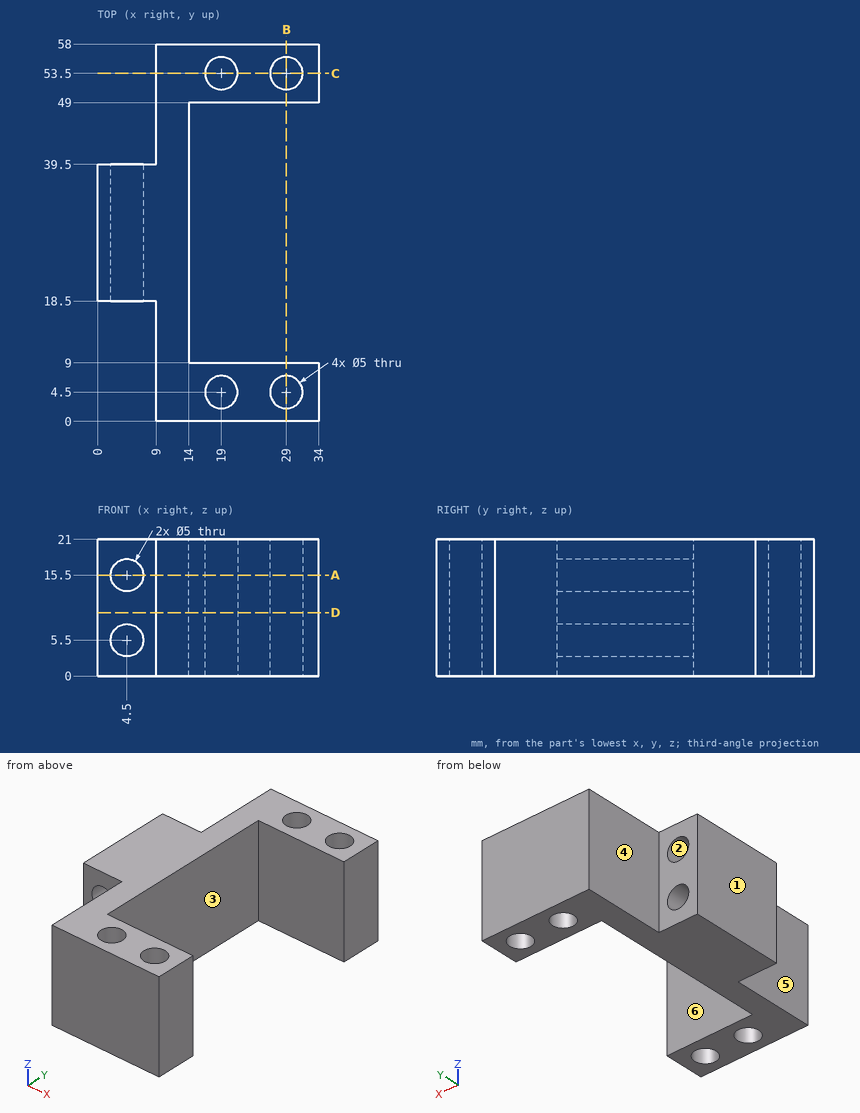
Check sheet for the drawn part. Datum: minimum x, y, z corner. Units: mm. A direction names the side the tool comes from. Round coordinates to 2 decimals unless told otherwise and drop trailing zeros. Order: outer loops, then holes, each group sorted by start corner. A loop starts at its lowest first (then second) coordinate and runs counter-clockwise, first axis right, second up. Notation, with made-up numbers: (22.25, 38.25) - (33.25, 38.25) arc R10 cw to (33.25, 48.25) - close; hole circle Ø8 at (-31.75, -24). An arc over 180 degrees is marked (long way). Use a Markdown table: item, result. Add a question column.
(1) Sectioned sample at D-D, the plane z = 9.75. Enter the section's corners in (x, y).
(2) Sectioned sample at A-A, the plane z = 15.5. Enter the section's corners in (x, y), and give its area (3 significant figures).
(3) Material ranges on line 1 along Z through (x, y) = (4.5, 28.5); line 2 along Z through (x, y) = (4, 27); line 3 along Y through (x, z) = (29.5, 12), recorded low to high. Write a range as [from, to].
(4) Sectioned sample at C-C, the plane y = 53.5. Enter the section's corners in (x, z).
(5) Depth check by flat-ended pin: pin 1 (6 mm diameter, centred on x = 4.5, z = 5.5, fed in from -Y); pin 2 (4 mm diameter, centred on y = 49, z = 14.5, fed in from -X); pin 3 (4 mm diameter, centred on x = 4.5, z = 15.5, fed in from -Y); pin 4 (7 mm diameter, centred on x = 2.5, z = 14, fed in from +Y). Enter the tip coordinate at first touch or a pass-through.
(6) Sectioned sample at B-B, the plane x = 29. Enter the section's corners in (y, z).
(7) Release check for a two-part mould opening along X. For the marked faces 1, 2 and 3 record: pulls with the +X half, pulls with the -X half, needs draft (parallel to the pull), parting line crosses it, or undercut.
(8) Tool access check on the marked faces 4, 5 and 6. Record the directions out of +Z, -Z, +X, -X, +Y, -Y that give a thin tool (end or side, any length) a straight path to the whole face; none if there is none.
Answers below:
| question | item | result |
|---|---|---|
| 1 | outline | (0, 18.5) - (9, 18.5) - (9, 0) - (34, 0) - (34, 9) - (14, 9) - (14, 49) - (34, 49) - (34, 58) - (9, 58) - (9, 39.5) - (0, 39.5) - close; hole circle Ø5 at (19, 4.5); hole circle Ø5 at (19, 53.5); hole circle Ø5 at (29, 4.5); hole circle Ø5 at (29, 53.5) |
| 2 | outline | (0, 18.5) - (2, 18.5) - (2, 39.5) - (0, 39.5) - close; (7, 18.5) - (9, 18.5) - (9, 0) - (34, 0) - (34, 9) - (14, 9) - (14, 49) - (34, 49) - (34, 58) - (9, 58) - (9, 39.5) - (7, 39.5) - close; hole circle Ø5 at (19, 4.5); hole circle Ø5 at (19, 53.5); hole circle Ø5 at (29, 4.5); hole circle Ø5 at (29, 53.5) |
| 2 | area | 655 mm² |
| 3 | line 1 | [0, 3], [8, 13], [18, 21] |
| 3 | line 2 | [0, 3.05], [7.95, 13.05], [17.95, 21] |
| 3 | line 3 | [0, 2.05], [6.95, 9], [49, 51.05], [55.95, 58] |
| 4 | outline | (9, 0) - (16.5, 0) - (16.5, 21) - (9, 21) - close; (21.5, 0) - (26.5, 0) - (26.5, 21) - (21.5, 21) - close; (31.5, 0) - (34, 0) - (34, 21) - (31.5, 21) - close |
| 5 | pin 1 | y = 18.5 |
| 5 | pin 2 | x = 9 |
| 5 | pin 3 | through |
| 5 | pin 4 | y = 39.5 |
| 6 | outline | (0, 0) - (2, 0) - (2, 21) - (0, 21) - close; (7, 0) - (9, 0) - (9, 21) - (7, 21) - close; (49, 0) - (51, 0) - (51, 21) - (49, 21) - close; (56, 0) - (58, 0) - (58, 21) - (56, 21) - close |
| 7 | face 1 | pulls with the -X half |
| 7 | face 2 | undercut |
| 7 | face 3 | pulls with the +X half |
| 8 | face 4 | +Z, -Z, -X, +Y |
| 8 | face 5 | +Z, -Z, -X, -Y |
| 8 | face 6 | +Z, -Z, +X |
